Input: part model. Units: mm. Frame: model coordinates. A direction names the side the tool comes from. Round coordinates to 2 decimals unless told otherwise and drop trailing zeros. Order: outer loops, then holes, each group sorted by start corner. A loop starts at its lowest first (then second) coordinate and runs counter-clockwise, first axis right, second up. Notation, with made-up numbers: (20, -9) -> (54, -9) arc R20 cw to (54, 24) -> close; hole circle Ø5 at (20.5, -8.5). An arc over 180 degrees is marked (long way). Use a Markdown table: item, result.
from build123d import *

# Parameters (mm, degrees)
SKETCH2_W           = 54.4
SKETCH2_H           = 16
BOSS_EXTRUDE1_DEPTH = 4
SKETCH3_W           = 2.3
SKETCH3_H           = 24
BOSS_EXTRUDE2_DEPTH = 54.4
SKETCH4_R           = 2.3
CUT_EXTRUDE1_DEPTH  = 45
CUT_EXTRUDE3_DEPTH  = 10
SKETCH5_R           = 8
CUT_EXTRUDE2_DEPTH  = 10
CUT_EXTRUDE4_DEPTH  = 10
SKETCH8_W           = 2.5
SKETCH8_H           = 10.25
BOSS_EXTRUDE3_DEPTH = 54.4
SKETCH9_W           = 2.5
SKETCH9_H           = 3.3
BOSS_EXTRUDE4_DEPTH = 10.25
CUT_EXTRUDE5_DEPTH  = 3.3


with BuildPart() as part:
    # Sketch2 → Boss-Extrude1 (new body)
    with BuildSketch(Plane(origin=(0, 0, 0), x_dir=(1, 0, 0), z_dir=(0, 1, 0))):
        Rectangle(SKETCH2_W, SKETCH2_H)
    extrude(amount=BOSS_EXTRUDE1_DEPTH)

    # Sketch3 → Boss-Extrude2 (add)
    with BuildSketch(Plane(origin=(27.2, 0, 0), x_dir=(0, 0, -1), z_dir=(1, 0, 0))):
        with Locations((-9.15, 12)):
            Rectangle(SKETCH3_W, SKETCH3_H)
    extrude(amount=-BOSS_EXTRUDE2_DEPTH)

    # Sketch4 → Cut-Extrude1 (cut)
    with BuildSketch(Plane(origin=(0, 4, 0), x_dir=(1, 0, 0), z_dir=(0, 1, 0))):
        with Locations((-13.5, 2.5)):
            Circle(SKETCH4_R)
        with Locations((13.5, 2.5)):
            Circle(SKETCH4_R)
    extrude(amount=-CUT_EXTRUDE1_DEPTH, mode=Mode.SUBTRACT)

    # Sketch6 → Cut-Extrude3 (cut)
    with BuildSketch(Plane.XY.offset(10.3)):
        with BuildLine():
            Line((-3.75, 7.85), (3.75, 7.85))
            ThreePointArc((3.75, 7.85), (5.3, 6.3), (3.75, 4.75))
            Line((3.75, 4.75), (-3.75, 4.75))
            ThreePointArc((-3.75, 4.75), (-5.3, 6.3), (-3.75, 7.85))
        make_face()
    extrude(amount=-CUT_EXTRUDE3_DEPTH, mode=Mode.SUBTRACT)

    # Sketch5 → Cut-Extrude2 (cut)
    with BuildSketch(Plane.XY.offset(10.3)):
        with Locations((-13.5, 14.25)):
            Circle(SKETCH5_R)
        with Locations((13.5, 14.25)):
            Circle(SKETCH5_R)
    extrude(amount=-CUT_EXTRUDE2_DEPTH, mode=Mode.SUBTRACT)

    # Sketch7 → Cut-Extrude4 (cut)
    with BuildSketch(Plane.XY.offset(10.3)):
        Polygon((-35.24269893, 14.25), (-13.5, 14.25), (-5.3, 6.3), (0, 6.5), (5.3, 6.3), (13.5, 14.25), (21.5, 14.25), (36.006358293, 14.25), (36.006358293, 27.887641337), (-35.24269893, 27.887641337), align=None)
    extrude(amount=-CUT_EXTRUDE4_DEPTH, mode=Mode.SUBTRACT)

    # Sketch8 → Boss-Extrude3 (add)
    with BuildSketch(Plane(origin=(27.2, 0, 0), x_dir=(0, 0, -1), z_dir=(1, 0, 0))):
        with Locations((-3.45, 9.125)):
            Rectangle(SKETCH8_W, SKETCH8_H)
    extrude(amount=-BOSS_EXTRUDE3_DEPTH)

    # Sketch9 → Boss-Extrude4 (add)
    with BuildSketch(Plane(origin=(0, 4, 0), x_dir=(1, 0, 0), z_dir=(0, 1, 0))):
        with Locations((-25.95, -6.35)):
            Rectangle(SKETCH9_W, SKETCH9_H)
        with Locations((25.95, -6.35)):
            Rectangle(SKETCH9_W, SKETCH9_H)
    extrude(amount=BOSS_EXTRUDE4_DEPTH)

    # Sketch10 → Cut-Extrude5 (cut)
    with BuildSketch(Plane.XY.offset(4.7)):
        Polygon((-27.2, 8.25), (-25.2, 8.25), (-27.2, 11.25), align=None)
        Polygon((27.2, 11.25), (27.2, 8.25), (25.2, 8.25), align=None)
    extrude(amount=CUT_EXTRUDE5_DEPTH, mode=Mode.SUBTRACT)


solid = part.part
1) Cut plane C-C on y = 1.25. Return loops of the section in (x, z), and give its area (3 significant figures).
Results found:
| item | result |
|---|---|
| outline | (-27.2, -8) -> (27.2, -8) -> (27.2, 10.3) -> (-27.2, 10.3) -> close; hole circle Ø4.6 at (-13.5, -2.5); hole circle Ø4.6 at (13.5, -2.5) |
| area | 962 mm² |
2) Pin query (flat end, axial travel): pin 1 Ø1 at (x, z) = (-6.5, 6.5) entering from +Y; pin 2 Ø1.6 at (x, y) = (-25.5, 10.5) entering from -Z; pin 3 Ø1.5 at (x, z) = (-3.5, 2) entering from +Y; pin 4 Ø3.5 at (x, z) = (-13.5, -2.5) entering from -Y. Return the tip coordinate at first contact, or that it passes through.
Results found:
| item | result |
|---|---|
| pin 1 | stops at y = 4 |
| pin 2 | stops at z = 2.2 |
| pin 3 | stops at y = 14.25 |
| pin 4 | passes through |
3) Cut plane A-A on z = -2.5. Return loops of the section in (x, y).
Results found:
| item | result |
|---|---|
| outline | (-27.2, 0) -> (-15.8, 0) -> (-15.8, 4) -> (-27.2, 4) -> close; (-11.2, 0) -> (11.2, 0) -> (11.2, 4) -> (-11.2, 4) -> close; (15.8, 0) -> (27.2, 0) -> (27.2, 4) -> (15.8, 4) -> close |
4) Line query: L1, parallel to X at y = 2, z = -2.5; L2, parallel to Z at x = 23, y = 11.75; L3, parallel to X at y = 13.75, z = 6. Output: solid intervals per line, ascending. Write a range as [from, to].
Results found:
| item | result |
|---|---|
| L1 | x = [-27.2, -15.8], [-11.2, 11.2], [15.8, 27.2] |
| L2 | z = [2.2, 4.7], [8, 10.3] |
| L3 | x = [-27.2, -24.7], [24.7, 27.2] |
5) Pull-direction query (Z, two-part tool) for faces 6 (the flat face through (-27, 9, 4.7)), 7 (the flat face through (0, 4, 10.3)), 8 (the flat face through (0, 14.25, 4)); classes: +Z half, -Z half, draft (parallel to the pull), parting line (faces both ways), or undercut.
Results found:
| item | result |
|---|---|
| face 6 | undercut |
| face 7 | +Z half |
| face 8 | draft |
6) Set-up query: faces 1 (the flat face through (0, 4, -3)), 2 (the flat face through (0, 4.75, 9)), 3 (the flat face through (0.3, 4.5, 8)), 4 (the flat face through (27, 9, 8)), 5 (the flat face through (-26.186, 9.729, 6.327)). Return all of +Z, -Z, +X, -X, +Y, -Y with unobstructed straight access to the full face (end or side cutting, diameter ignored); none if empty.
Results found:
| item | result |
|---|---|
| face 1 | -Z, +X, -X, +Y |
| face 2 | +Z, +Y |
| face 3 | +Y |
| face 4 | +X |
| face 5 | -X |
7) Cut plane B-B on x = 23. Return loops of the section in (y, z).
Results found:
| item | result |
|---|---|
| outline | (0, -8) -> (4, -8) -> (4, 2.2) -> (14.25, 2.2) -> (14.25, 4.7) -> (4, 4.7) -> (4, 8) -> (14.25, 8) -> (14.25, 10.3) -> (0, 10.3) -> close |
8) Cut plane D-D on x = 13.5. Return loops of the section in (y, z), and give its area (3 significant figures).
Results found:
| item | result |
|---|---|
| outline | (0, -8) -> (4, -8) -> (4, -4.8) -> (0, -4.8) -> close; (0, -0.2) -> (4, -0.2) -> (4, 2.2) -> (14.25, 2.2) -> (14.25, 4.7) -> (4, 4.7) -> (4, 8) -> (6.25, 8) -> (6.25, 10.3) -> (0, 10.3) -> close |
| area | 85.6 mm² |
